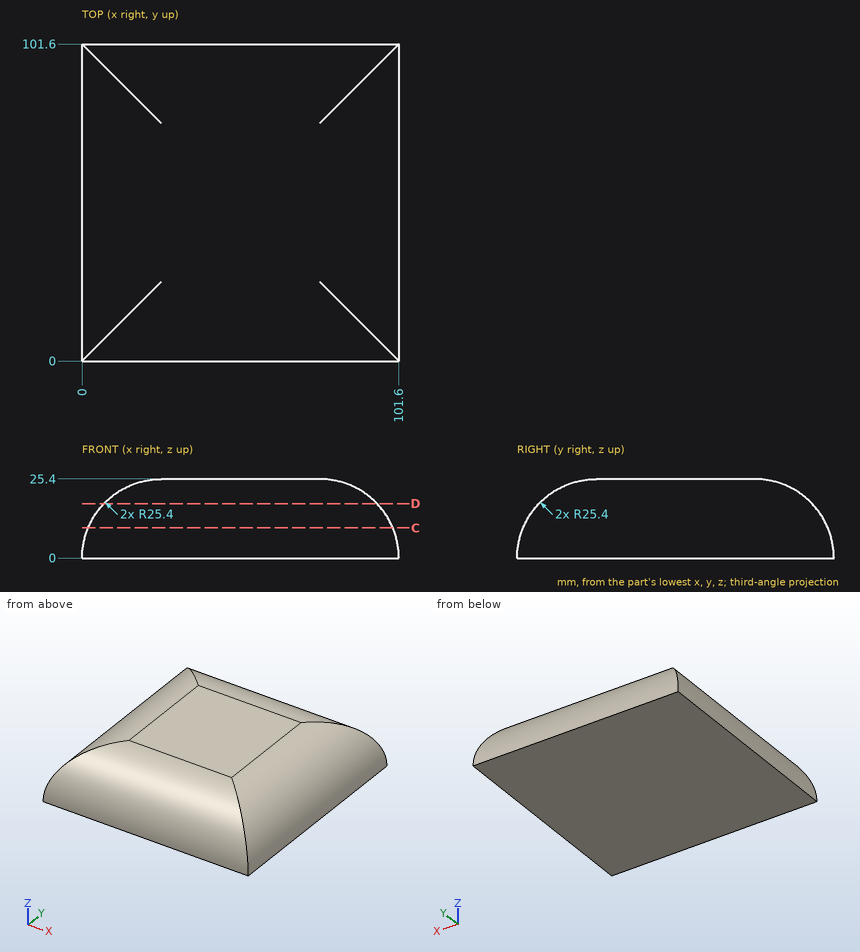
Verification items for this drawing (mm, ordinates from the low corner). Coordinates: 2 decimals unless noted, no trailing zeros. Write each loop counter-clockwise with the first axis right and the second up, starting at its lowest first coordinate (ties: lowest second). Pieces come first, ordered by that corner, then holes. Notation, with made-up numbers: M 12.25,18 L 51.25,18 A18 cw 51.25,33 Z; hole C 12,-21.5 d3. An arc over 180 degrees is marked long. Use CSV: the item, a comma, the result in double quotes.
Q1. Thickness scan on line 1 along X through (y, z) = (5, 1); line 2 along Z through (x, y) = (33.5, 7); line 3 along Y through (x, z) = (36, 21). Record the ranges inside material, lowest first. Write a range as [from, to].
Computed values:
line 1,"[0.02, 101.58]"
line 2,"[0, 17.51]"
line 3,"[11.11, 90.49]"
Q2. Go/stop test with flat-tipped pins: P1, Ø6, axis at x = 45.5, z = 20, coming from the -Y side; P2, Ø1.5, axis at x = 35.5, y = 24, coming from the +Z side; P3, Ø1, axis at y = 31, z = 14.5, coming from the +X side. Record where each tip stops, or that it passes through.
Computed values:
P1,"y = 6.53"
P2,"z = 25.39"
P3,"x = 97.39"
Q3. Section check D-D, the plane z = 17.5. Enter the section's corners in (x, y), and give its area (3 significant figures).
Computed values:
outline,"M 6.99,6.99 L 94.61,6.99 L 94.61,94.61 L 6.99,94.61 Z"
area,"7,680 mm²"
Q4. Section check C-C, the plane z = 9.75. Enter the section's corners in (x, y).
Computed values:
outline,"M 1.95,1.95 L 99.65,1.95 L 99.65,99.65 L 1.95,99.65 Z"
